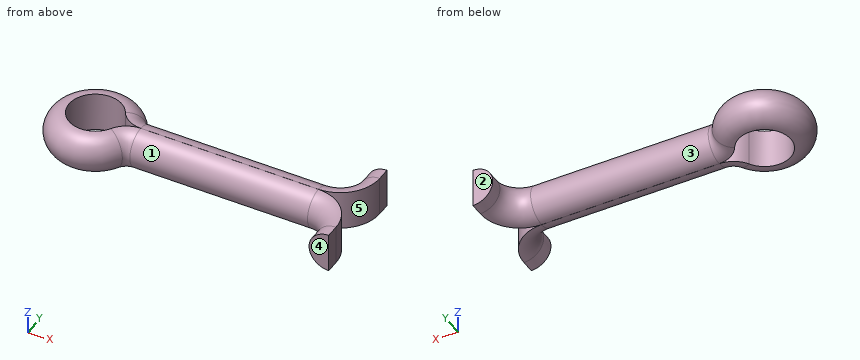
from build123d import *


with BuildPart() as part:
    # Sweep1: sweep along a path in Sketch1
    with BuildLine(Plane.XY) as sweep1_path:
        Line((20, 4), (20, 3))
        ThreePointArc((20, 3), (19.121320344, 0.878679656), (17, 0))
        Line((17, 0), (3.464101615, 0))
        ThreePointArc((3.464101615, 0), (2.464101615, 0.267949192), (1.732050808, 1))
        ThreePointArc((1.732050808, 1), (-1.999997913, 0.002889164), (1.729154418, -1.005))
        ThreePointArc((1.729154418, -1.005), (2.460811968, -0.276506418), (3.458308835, -0.01))
        Line((3.458308835, -0.01), (17, -0.01))
        ThreePointArc((17, -0.01), (19.121320344, -0.888679656), (20, -3.01))
        Line((20, -3.01), (20, -4.01))
    # Sketch3 → Sweep1 (sweep)
    with BuildSketch(Plane(origin=(20, 4, 0), x_dir=(1, 0, 0), z_dir=(0, 1, 0))):
        with BuildLine():
            Line((0, 1.5), (0, -1.5))
            ThreePointArc((0, -1.5), (-1.5, 0), (0, 1.5))
        make_face()
    sweep(path=sweep1_path.line)


solid = part.part
Read the model definition and answer for the solid it produces. Units are mm, in the model's axes. Face numbers are marked on the shaded views. A direction names the side the tool comes from. Give positions to 0.01 mm unless a question says otherwise; leave off trailing zeros. Write each loop counter-clockwise with the first axis right and the second up, starting at its lowest first coordinate (ties: lowest second). Pieces come first, ordered by that corner, then holes. Notation, with made-up numbers: (62.25, 26) - (86.25, 26) arc R16 ccw to (86.25, 52) - close; hole circle Ø8 at (49.25, -19.75). An arc over 180 degrees is marked (long way). Return JSON: item names as keys, results as strings.
Q1. Consider line 1 along Y through (x, z) = (0, 0); line 2 along X through (y, z) = (1.5, 0.75); line 3 along X through (y, z) = (1, -0.7). Determine where each line is inside the solid, lowest interval first. Write a range as [from, to].
Reply:
{"line 1": "[-3.5, -2], [2, 3.5]", "line 2": "[-2.94, -1.32], [1.32, 2.97], [17.8, 19.6]", "line 3": "[-3.17, -1.73], [1.73, 19.24]"}
Q2. A cutting plane is placed at B-B, the plane x = 5. Determine the outline of the cut face in (y, z), and give its area (3 significant figures).
Reply:
{"outline": "(-0.01, -1.5) - (-0.01, 1.5) arc R1.5 ccw to start; (0, -1.5) arc R1.5 ccw to (0, 1.5) - close", "area": "7.07 mm²"}
Q3. For a pull along Y with two mould halves and no side action, classify the marked faces 3, 4 and 5 as released by +Y, released by -Y, zero draft, split by the parting line, or undercut.
Reply:
{"face 3": "released by +Y", "face 4": "released by -Y", "face 5": "undercut"}
Q4. A cutting plane is placed at A-A, the plane z = 0.5. Determine the outline of the cut face in (x, y) (3 decimals).
Reply:
{"outline": "(1.729, -1.005) arc R2 cw (long way) to (1.732, 1) arc R2 ccw to (3.464, 0) - (17, 0) arc R3 ccw to (20, 3) - (20, 4) - (18.586, 4) - (18.586, 3) arc R1.586 cw to (17, 1.414) - (3.464, 1.414) arc R0.586 cw to (2.957, 1.707) arc R3.414 ccw (long way) to (2.952, -1.716) arc R0.586 cw to (3.458, -1.424) - (17, -1.424) arc R1.586 cw to (18.586, -3.01) - (18.586, -4.01) - (20, -4.01) - (20, -3.01) arc R3 ccw to (17, -0.01) - (3.458, -0.01) arc R2 ccw to start"}
Q5. For the marked faces 1 and 2, determine the directions among +Z, -Z, +X, -X, +Y, -Y from which every point of the face is accessible in a straight line to the end or side of a thin tool.
Reply:
{"face 1": "-Y", "face 2": "+Z, -Z, +X, -X, +Y"}
Q6. Given P1, Ø1.5, axis at x = 0, y = -0.5, coming from the +Z side; P2, Ø1.5, axis at y = -2, z = 1, coming from the +X side; P3, Ø1, axis at x = 8.5, z = -1, coming from the +Y side, each flat-ended and moving along its own axis, determine where each tip first touches the part or whether it passes through.
Reply:
{"P1": "through", "P2": "x = 19.99", "P3": "y = 1.41"}
